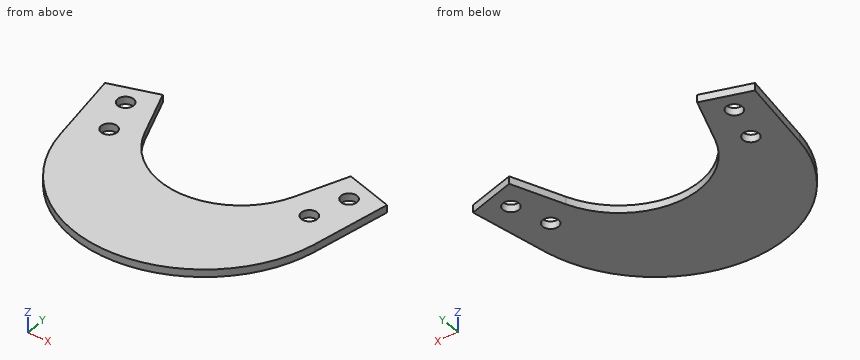
from build123d import *

# Parameters (mm, degrees)
SKETCH1_R           = 1.6
BOSS_EXTRUDE1_DEPTH = 1.5


with BuildPart() as part:
    # Sketch1 → Boss-Extrude1 (new body)
    with BuildSketch(Plane.XY):
        with BuildLine():
            Line((25.85974293, -14.554976912), (28.663386119, 1.32487132))
            Line((28.663386119, 1.32487132), (19.108746057, 4.275947949))
            Line((19.108746057, 4.275947949), (15.138453004, -5.904104582))
            ThreePointArc((15.138453004, -5.904104582), (0, -16.249037211), (-15.138453004, -5.904104582))
            Line((-15.138453004, -5.904104582), (-19.108746057, 4.275947949))
            Line((-19.108746057, 4.275947949), (-28.663386119, 1.32487132))
            Line((-28.663386119, 1.32487132), (-25.85974293, -14.554976912))
            ThreePointArc((-25.85974293, -14.554976912), (0, -36.249037211), (25.85974293, -14.554976912))
        make_face()
        with Locations(Location((-20.344774133, -8.665158441, 0), (0, 0, 180))):
            Circle(SKETCH1_R, mode=Mode.SUBTRACT)
        with Locations(Location((-22.705635436, -1.021446391, 0), (0, 0, 180))):
            Circle(SKETCH1_R, mode=Mode.SUBTRACT)
        with Locations((22.705635436, -1.021446391)):
            Circle(SKETCH1_R, mode=Mode.SUBTRACT)
        with Locations((20.344774133, -8.665158441)):
            Circle(SKETCH1_R, mode=Mode.SUBTRACT)
    extrude(amount=BOSS_EXTRUDE1_DEPTH)


solid = part.part
Geometry: final body of the model. Coordinates: model frame, mm. Round coordinates to 2 decimals unless told otherwise and drop trailing zeros. Loops run counter-clockwise (first coordinate to the right, second up) from the corner with the lowest first, then second, coordinate; pieces in that order, holes last.
Q1. Section A-A on y = -6.5. Return loops of the section in (x, z).
Q2. Section C-C on z = 1.2. Return loops of the section in (x, y), plus the area to 3 significant figures.
Q3. Section B-B on x = 23. Return loops of the section in (y, z), plus the area to 3 significant figures.
Q4. Section D-D on x = 2. Return loops of the section in (y, z), plus the area to 3 significant figures.
Q5. Material intervals for L1, parallel to X at y = -28, z = 0.65; L2, parallel to Y at x = -20.5, z = 0.45; L3, parallel to X at y = -6, z = 0.65, sorted ascending.
Evaluation:
1. outline: (-27.28, 0) - (-14.89, 0) - (-14.89, 1.5) - (-27.28, 1.5) - close; (14.89, 0) - (27.28, 0) - (27.28, 1.5) - (14.89, 1.5) - close
2. outline: (-28.66, 1.32) - (-25.86, -14.55) arc R26.26 ccw to (25.86, -14.55) - (28.66, 1.32) - (19.11, 4.28) - (15.14, -5.9) arc R16.25 cw to (-15.14, -5.9) - (-19.11, 4.28) - close; hole circle Ø3.2 at (-22.71, -1.02); hole circle Ø3.2 at (-20.34, -8.67); hole circle Ø3.2 at (20.34, -8.67); hole circle Ø3.2 at (22.71, -1.02)
2. area: 1,240 mm2
3. outline: (-22.66, 0) - (-2.59, 0) - (-2.59, 1.5) - (-22.66, 1.5) - close; (0.55, 0) - (3.07, 0) - (3.07, 1.5) - (0.55, 1.5) - close
3. area: 33.9 mm2
4. outline: (-36.17, 0) - (-16.13, 0) - (-16.13, 1.5) - (-36.17, 1.5) - close
4. area: 30.1 mm2
5. L1: x = -19.11 to 19.11
5. L2: y = -26.4 to -10.26, -7.07 to 3.85
5. L3: x = -27.37 to -15.1, 15.1 to 27.37
